Could you check a few things on this model? Use its own coordinates, in mm. A direction names the side the tool comes from. Round coordinates to 2 decimals unless told otherwise and drop trailing zeros. Loops run counter-clockwise (first coordinate to the right, second up) from the corner with the lowest first, then second, coordinate; pieces in that order, holes last. Notation, with made-up numbers: M 34,62 L 53,62 A23 ccw 53,92 Z; hole C 48.25,68 d1. An arc over 180 degrees is marked long. Return JSON: item names as keys, results as strings. Group by question number.
```python
from build123d import *

# Parameters (mm, degrees)
SKETCH2_W          = 22
SKETCH2_H          = 21
SKETCH2_W_2        = 20
SKETCH2_H_2        = 5.8
CUT_EXTRUDE1_DEPTH = 3.2


with BuildPart() as part:
    # Sketch1 → Revolve1 (revolve)
    with BuildSketch(Plane.XY):
        Polygon((0, 9.8), (0, 6), (10.2, 6), (10.2, 10), (0.2, 10), align=None)
    revolve(axis=Axis((10.2, 0, 0), (-1, 0, 0)))

    # Sketch2 → Cut-Extrude1 (cut)
    with BuildSketch(Plane(origin=(10.2, 0, 0), x_dir=(0, 0, -1), z_dir=(1, 0, 0))):
        Rectangle(SKETCH2_W, SKETCH2_H)
        Rectangle(SKETCH2_W_2, SKETCH2_H_2, mode=Mode.SUBTRACT)
    extrude(amount=-CUT_EXTRUDE1_DEPTH, mode=Mode.SUBTRACT)

    # Sketch3 → Cut-Revolve1 (revolve, cut)
    with BuildSketch(Plane(origin=(3.4, 0, 0), x_dir=(0, 0, -1), z_dir=(1, 0, 0))):
        Polygon((-10, 0), (-10, 2), (-9.621, 1.621), (0, 1.621), (0, 0), align=None)
    revolve(axis=Axis((3.4, 0, 0), (0, 0, 1)), mode=Mode.SUBTRACT)

    # Sketch4 → Cut-Revolve2 (revolve, cut)
    with BuildSketch(Plane(origin=(3.4, 0, 0), x_dir=(0, 0, -1), z_dir=(1, 0, 0))):
        Polygon((0, -10), (-2, -10), (-1.621, -9.621), (-1.621, 0), (0, 0), align=None)
    revolve(axis=Axis((3.4, 0, 0), (0, -1, 0)), mode=Mode.SUBTRACT)


solid = part.part
```
1. If we section it at C-C, the plane x = 3.4: Please give me the cut outline in (y, z), then the cut area to 3 significant figures.
2. If we section it at B-B, the plane y = 0: Please give me the cut outline in (x, z), then the cut area to 3 significant figures.
3. On a 3-axis mill with a long thin cutter (end or side, diameter ignored), from which of +Z, -Z, +X, -X, +Y, -Y can I reach the whole of each face in a straight line? I mean faces 1 (the face through (2.913, -7.669, 1.546)), 2 (the face through (9, -2.9, -7)), 3 (the face through (4.04, 5.54, 2.3)), 4 (the face through (7, 6.5, 0.1)). Say none if no direction works.
4. If we section it at D-D, the plane x = 6.5: Please give me the cut outline in (y, z).
5. I need wall thicknesses on probe 1 along X at (y, z) = (-7.35, 0); probe 2 along Z at (x, y) = (3.4, -8); probe 3 along Y at (x, z) = (9.5, 8). Which ranges of each line are inside material? Lowest first, please.
6. If we section it at A-A, the plane z = 0: Please give me the cut outline in (x, y), then the cut area to 3 significant figures.
7. I'm going to push flat-ended pins straight in: pin 1 Ø8 at (y, z) = (5, 0) entering from -X; pin 2 Ø8 at (y, z) = (5.5, -2) entering from +X; pin 3 Ø1 at (x, z) = (8.5, -8.5) entering from +Y; pin 4 Ø1 at (x, y) = (9, 5.5) entering from -Z. Where does each tip first touch, or does it pass through?
8. We'd pull the mould along X, two halves only. Please class faces 5 (the face through (2.913, 1.546, 7.669)), 6 (the face through (9, 2.9, 7)), 7 (the face through (7, -6.4, 0.1)), 8 (the face through (0, 4.2, -4.5)): +X half, -X half, draft (parallel to the pull), parting line (faces both ways), or undercut.
Geometry results:
{
 "1": {"outline": "M -9.83,-1.83 A10 ccw long 1.83,9.83 L 1.62,9.62 L 1.62,5.78 A6 cw long -5.78,-1.62 L -9.62,-1.62 Z; M -9.83,1.83 L -9.62,1.62 L -5.78,1.62 A6 cw -1.62,5.78 L -1.62,9.62 L -1.83,9.83 A10 ccw Z", "area": "175 mm^2"},
 "2": {"outline": "M 0,-9.8 L 0.2,-10 L 10.2,-10 L 10.2,-6 L 0,-6 Z; M 0,6 L 1.78,6 L 1.78,9.62 L 1.4,10 L 0.2,10 L 0,9.8 Z; M 5.02,6 L 10.2,6 L 10.2,10 L 5.4,10 L 5.02,9.62 Z", "area": "68.4 mm^2"},
 "3": {"face 1": "-Y", "face 2": "+Z, -Z, +X, -Y", "face 3": "+X, -X", "face 4": "+Z, -Z, +X, +Y"},
 "4": {"outline": "C 0,0 d20; hole C 0,0 d12"},
 "5": {"probe 1": "0 to 1.78, 5.02 to 7", "probe 2": "-6 to -1.62, 1.62 to 6", "probe 3": "-2.9 to 2.9"},
 "6": {"outline": "M 0,-9.8 L 0.2,-10 L 1.4,-10 L 1.78,-9.62 L 1.78,-6 L 0,-6 Z; M 0,6 L 7,6 L 7,10 L 0.2,10 L 0,9.8 Z; M 5.02,-9.62 L 5.4,-10 L 7,-10 L 7,-6 L 5.02,-6 Z", "area": "42.8 mm^2"},
 "7": {"pin 1": "x = 0", "pin 2": "x = 7", "pin 3": "y = 2.9", "pin 4": "through"},
 "8": {"face 5": "undercut", "face 6": "draft", "face 7": "+X half", "face 8": "-X half"}
}
